Here's the drawing with two shaded views (mm, measured from the low corner). I have some questions. A direction names the side the tool comes from. Coordinates: 2 decimals unless noted, no trailing zeros. Write each loop counter-clockwise with the first axis right and the second up, starting at its lowest first coordinate (ties: lowest second). Pieces come first, ordered by that corner, then holes.
Item 1: If I drill on probe 1 along Z at (x, y) = (80.5, 116); probe 2 along X at (y, z) = (46.5, 20); probe 3 along Y at (x, z) = (76.5, 43.5), over which ranges is the centre line in solid material (lowest first)?
Item 2: I want a section at B-B on x = 30. Please give me the cut outline in (y, z).
Item 3: I want a section at C-C on z = 25.5. Please give me the cut outline in (x, y), then the cut area to 3 significant figures.
Item 4: Which directions (+Z, -Z, +X, -X, +Y, -Y) give clear straight access to the entire face, cutting with the end or side of a thin tool? Please do the marked faces 1, 2, 3 and 4.
Item 5: I want a section at D-D on x = 70.5. Please give me the cut outline in (y, z).
Item 6: For P1, Ø14.5, axis at x = 78.5, z = 35, coming from the +Y side; P2, Ø24.5, axis at x = 93.5, z = 32.5, coming from the -Y side; P3, Ø8.5, axis at y = 57, z = 25.5, coming from the -X side, each with a flat end and sliding along its axis, tell me the tip position at first contact or that it passes through.
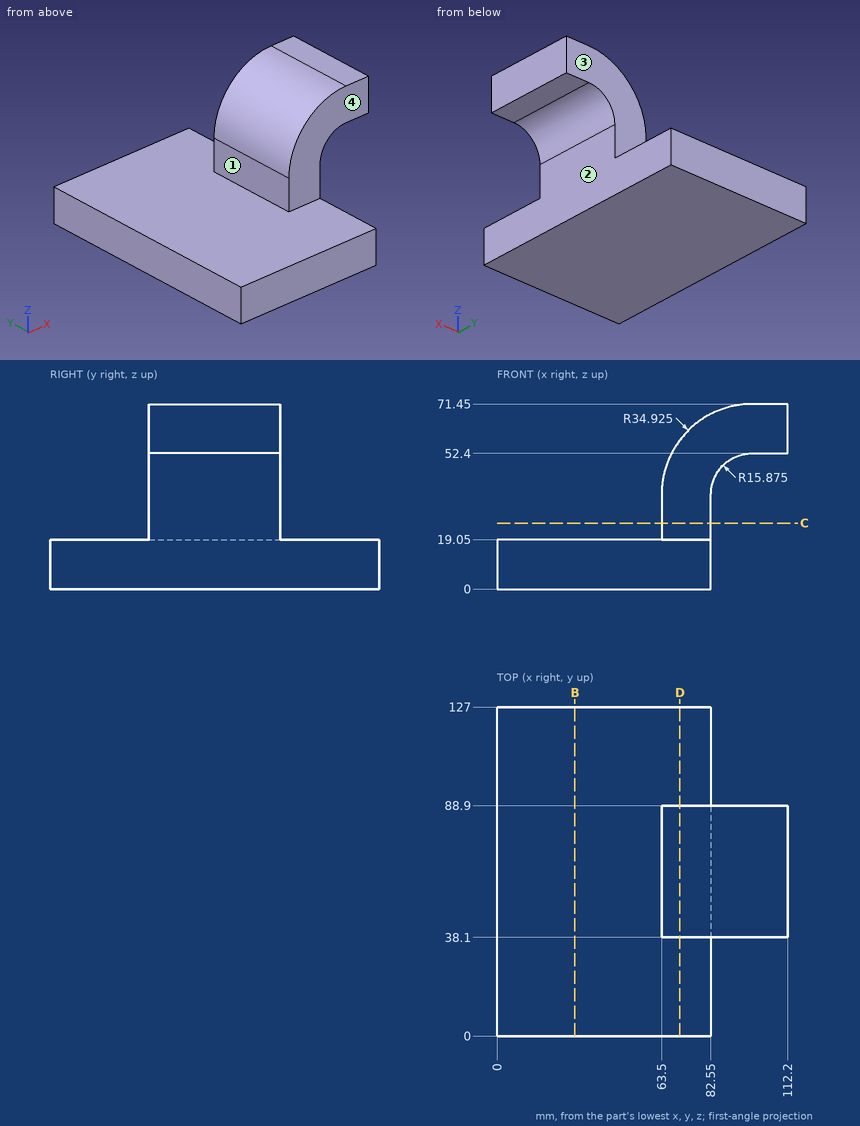
Response values:
1. probe 1: z = 0 to 19.05
1. probe 2: x = 63.5 to 82.55
1. probe 3: y = 38.1 to 88.9
2. outline: (0, 0) - (127, 0) - (127, 19.05) - (0, 19.05) - close
3. outline: (63.5, 38.1) - (82.55, 38.1) - (82.55, 88.9) - (63.5, 88.9) - close
3. area: 968 mm2
4. face 1: +Z, -X, +Y, -Y
4. face 2: -Z, +X, +Y, -Y
4. face 3: +Z, +X, -X, +Y
4. face 4: +Z, +X, -X, -Y
5. outline: (0, 0) - (127, 0) - (127, 19.05) - (88.9, 19.05) - (88.9, 57.5) - (38.1, 57.5) - (38.1, 19.05) - (0, 19.05) - close
6. P1: stops at y = 88.9
6. P2: stops at y = 38.1
6. P3: stops at x = 63.5
